Geometry check sheet. Reference: the model listing, model coordinates, mm. Round coordinates to 2 decimals unless told otherwise and drop trailing zeros. Write each loop counter-clockwise with the first axis right and the second up, starting at its lowest first coordinate (ties: lowest second). Pieces come first, ordered by that corner, then holes. Notation, with made-up numbers: M -33.5,-4.75 L -21.5,-4.75 A19 ccw -21.5,16.25 Z; hole C -31,4 d6. An arc over 180 degrees is marked long. Put each result on its own line as item: value. Start each with the question number.
(1) Material ranges on probe 1 along X at (y, z) = (1.25, -98.42) (3 decimals); probe 2 along Z at (x, y) = (74.3, 0.4) (3 decimals), recorded low to high.
(2) Gauge pin test, flat ends, axial feed: pin 1 (3 mm diameter, centred on x = 63.5, z = -18, fed in from -Y); pin 2 (3 mm diameter, centred on x = 140.33, z = -3.815, fed in from -Y). Record the tip position at first contact, or that the pin passes through.
(3) Section check A-A on x = 140.33. Record the cut outline in (y, z) (3 decimals), then the cut area to 3 significant figures.
from build123d import *

# Parameters (mm, degrees)
SKETCH1_W           = 144.145
SKETCH1_H           = 102.235
SKETCH1_R           = 1.7526
BOSS_EXTRUDE1_DEPTH = 1.6
SKETCH2_R           = 0.5
CUT_EXTRUDE1_DEPTH  = 2.6


with BuildPart() as part:
    # Sketch1 → Boss-Extrude1 (new body)
    with BuildSketch(Plane(origin=(0, 0, 0), x_dir=(1, 0, 0), z_dir=(0, 1, 0))):
        with Locations((72.0725, 51.1175)):
            Rectangle(SKETCH1_W, SKETCH1_H)
        with Locations((3.815, 98.42)):
            Circle(SKETCH1_R, mode=Mode.SUBTRACT)
        with Locations((140.33, 98.42)):
            Circle(SKETCH1_R, mode=Mode.SUBTRACT)
        with Locations((140.33, 3.815)):
            Circle(SKETCH1_R, mode=Mode.SUBTRACT)
        with Locations((3.815, 3.815)):
            Circle(SKETCH1_R, mode=Mode.SUBTRACT)
    extrude(amount=BOSS_EXTRUDE1_DEPTH)

    # Sketch2 → Cut-Extrude1 (cut, through all)
    with BuildSketch(Plane(origin=(0, 1.6, 0), x_dir=(1, 0, 0), z_dir=(0, 1, 0))):
        with Locations((36.2, 1.9)):
            Circle(SKETCH2_R)
        with Locations((38.74, 1.9)):
            Circle(SKETCH2_R)
        with Locations((41.28, 1.9)):
            Circle(SKETCH2_R)
        with Locations((43.82, 1.9)):
            Circle(SKETCH2_R)
        with Locations((46.36, 1.9)):
            Circle(SKETCH2_R)
        with Locations((48.9, 1.9)):
            Circle(SKETCH2_R)
        with Locations((51.44, 1.9)):
            Circle(SKETCH2_R)
        with Locations((53.98, 1.9)):
            Circle(SKETCH2_R)
        with Locations((56.52, 1.9)):
            Circle(SKETCH2_R)
        with Locations((59.06, 1.9)):
            Circle(SKETCH2_R)
        with Locations((61.6, 1.9)):
            Circle(SKETCH2_R)
        with Locations((64.14, 1.9)):
            Circle(SKETCH2_R)
        with Locations((66.68, 1.9)):
            Circle(SKETCH2_R)
        with Locations((69.22, 1.9)):
            Circle(SKETCH2_R)
        with Locations((71.76, 1.9)):
            Circle(SKETCH2_R)
        with Locations((74.3, 1.9)):
            Circle(SKETCH2_R)
        with Locations((76.84, 1.9)):
            Circle(SKETCH2_R)
        with Locations((79.38, 1.9)):
            Circle(SKETCH2_R)
        with Locations((81.92, 1.9)):
            Circle(SKETCH2_R)
        with Locations((84.46, 1.9)):
            Circle(SKETCH2_R)
        with Locations((87, 1.9)):
            Circle(SKETCH2_R)
    extrude(amount=-CUT_EXTRUDE1_DEPTH, mode=Mode.SUBTRACT)


solid = part.part
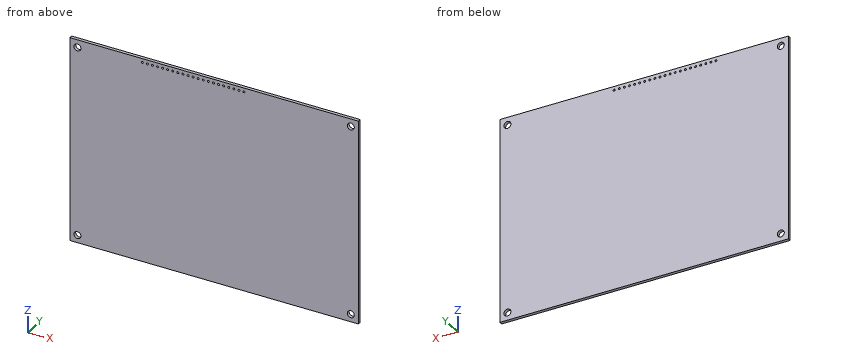
Answers follow:
1. probe 1: x = 0 to 2.062, 5.568 to 138.577, 142.083 to 144.145
1. probe 2: z = -102.235 to -2.4, -1.4 to 0
2. pin 1: stops at y = 0
2. pin 2: passes through
3. outline: M 0,-102.235 L 1.6,-102.235 L 1.6,-100.173 L 0,-100.173 Z; M 0,-96.667 L 1.6,-96.667 L 1.6,-5.568 L 0,-5.568 Z; M 0,-2.062 L 1.6,-2.062 L 1.6,0 L 0,0 Z
3. area: 152 mm^2
